Source: CAD feature listing. Evaluate the final solid. Frame: model axes, mm. A direction names the side the tool comes from. Give positions to 0.01 mm unless a question says otherwise; leave off trailing zeros. Loops run counter-clockwise (first coordinate to the right, second up) from the corner with the lowest first, then second, coordinate; pieces in that order, holes last. Notation, with made-up numbers: M 73,66 L 104,66 A10 ccw 104,78 Z; hole C 47,38 d8. An arc over 180 degrees is marked long. Put each result on its own line as item: value.
from build123d import *

# Parameters (mm, degrees)
SALIENTE_EXTRUIR1_DEPTH = 40
CORTAR_EXTRUIR4_DEPTH   = 10
CORTAR_EXTRUIR5_DEPTH   = 10
CORTAR_EXTRUIR6_DEPTH   = 2
CROQUIS8_R              = 1.5
CORTAR_EXTRUIR7_DEPTH   = 42
CROQUIS9_R              = 1.5
CORTAR_EXTRUIR8_DEPTH   = 42


with BuildPart() as part:
    # Croquis2 → Saliente-Extruir1 (new body)
    with BuildSketch(Plane.XY):
        Polygon((0, 26), (3, 26), (3, 4), (15, 4), (15, 0), (0, 0), align=None)
    extrude(amount=SALIENTE_EXTRUIR1_DEPTH)

    # Croquis6 → Cortar-Extruir4 (cut)
    with BuildSketch(Plane(origin=(3, 0, 0), x_dir=(0, 0, -1), z_dir=(1, 0, 0))):
        with BuildLine():
            Line((-40, 4), (-43.463242579, 10.305944429))
            Line((-43.463242579, 10.305944429), (-46.103119836, 28.990848346))
            Line((-46.103119836, 28.990848346), (-47.186653475, 36.660038985))
            Line((-47.186653475, 36.660038985), (8.796856155, 26.447825939))
            Line((8.796856155, 26.447825939), (6.381141064, 12.03440645))
            Line((6.381141064, 12.03440645), (0, 4))
            ThreePointArc((0, 4), (-20, 24), (-40, 4))
        make_face()
    extrude(amount=-CORTAR_EXTRUIR4_DEPTH, mode=Mode.SUBTRACT)

    # Croquis5 → Cortar-Extruir5 (cut)
    with BuildSketch(Plane(origin=(0, 4, 0), x_dir=(1, 0, 0), z_dir=(0, 1, 0))):
        with BuildLine():
            Line((15, -12), (15, -28))
            ThreePointArc((15, -28), (11.485281374, -36.485281374), (3, -40))
            Line((3, -40), (17.00840725, -44.81222058))
            Line((17.00840725, -44.81222058), (27.206798155, -5.039954665))
            Line((27.206798155, -5.039954665), (15.87267332, 7.755192399))
            Line((15.87267332, 7.755192399), (3, 0))
            ThreePointArc((3, 0), (11.485281374, -3.514718626), (15, -12))
        make_face()
    extrude(amount=-CORTAR_EXTRUIR5_DEPTH, mode=Mode.SUBTRACT)

    # Croquis7 → Cortar-Extruir6 (cut)
    with BuildSketch(Plane(origin=(0, 4, 0), x_dir=(1, 0, 0), z_dir=(0, 1, 0))):
        Polygon((7.9, -3.651368439), (5, -5.325684219), (5, -8.674315781), (7.9, -10.348631561), (10.8, -8.674315781), (10.8, -5.325684219), align=None)
        Polygon((5, -31.325684219), (5, -34.674315781), (7.9, -36.348631561), (10.8, -34.674315781), (10.8, -31.325684219), (7.9, -29.651368439), align=None)
    extrude(amount=-CORTAR_EXTRUIR6_DEPTH, mode=Mode.SUBTRACT)

    # Croquis8 → Cortar-Extruir7 (cut)
    with BuildSketch(Plane(origin=(0, 2, 0), x_dir=(1, 0, 0), z_dir=(0, 1, 0))):
        with Locations(Location((7.9, -7, 0), (0, 0, 270))):
            Circle(CROQUIS8_R)
    extrude(amount=-CORTAR_EXTRUIR7_DEPTH, mode=Mode.SUBTRACT)

    # Croquis9 → Cortar-Extruir8 (cut)
    with BuildSketch(Plane(origin=(0, 2, 0), x_dir=(1, 0, 0), z_dir=(0, 1, 0))):
        with Locations(Location((7.9, -33, 0), (0, 0, 180))):
            Circle(CROQUIS9_R)
    extrude(amount=-CORTAR_EXTRUIR8_DEPTH, mode=Mode.SUBTRACT)


solid = part.part
1. Section query B-B (z = 8). Output: boundary loops of the cut face in (x, y), plus the area to 3 significant figures.
Found:
outline: M 0,0 L 6.78,0 L 6.78,2 L 5,2 L 5,4 L 3,4 L 3,20 L 0,20 Z; M 9.02,0 L 14.31,0 L 14.31,4 L 10.8,4 L 10.8,2 L 9.02,2 Z
area: 89.2 mm^2
2. Section query A-A (y = 3.5). Output: boundary loops of the cut face in (x, z).
Found:
outline: M 0,0 L 3,0 A12 ccw 15,12 L 15,28 A12 ccw 3,40 L 0,40 Z; hole M 5,5.33 L 7.9,3.65 L 10.8,5.33 L 10.8,8.67 L 7.9,10.35 L 5,8.67 Z; hole M 5,31.33 L 7.9,29.65 L 10.8,31.33 L 10.8,34.67 L 7.9,36.35 L 5,34.67 Z
3. Draft query along Z for faces 4 (the flat face through (8, 0, 20)), 5 (the flat face through (9.37, 3.01, 30.5)), 6 (the cylindrical face through (11.58, 2.03, 36.39)). Return one class per face: pulls with the +Z half, pulls with the -Z half, needs draft (parallel to the pull), parting line crosses it, or undercut.
Found:
face 4: needs draft
face 5: undercut
face 6: pulls with the +Z half
4. Section query D-D (x = 6). Output: boundary loops of the cut face in (y, z), plus the area to 3 significant figures.
Found:
outline: M 0,0.38 L 4,0.38 L 4,4.75 L 2,4.75 L 2,9.25 L 4,9.25 L 4,30.75 L 2,30.75 L 2,35.25 L 4,35.25 L 4,39.62 L 0,39.62 Z
area: 139 mm^2
5. Section query C-C (y = 16). Output: boundary loops of the cut face in (x, z).
Found:
outline: M 0,4 L 3,4 L 3,36 L 0,36 Z
6. Contact query for flat-ended pins moving along their axis: P1, Ø6.5, axis at x = 7.5, z = 31.5, coming from the +Y side; P2, Ø1, axis at y = 3.5, z = 7.5, coming from the +X side; P3, Ø4, axis at x = 7.9, z = 33, coming from the +Y side; P4, Ø1.5, axis at x = 4, y = 18.5, coming from the -Z side. Output: stop coordinate, or through.
Found:
P1: y = 4
P2: x = 14.31
P3: y = 2
P4: through
7. Material intervals for line 1 (Y direction, x = 6.25, z = 31); line 2 (X direction, y = 2.5, z = 30); line 3 (X direction, y = 12, z = 35), sorted ascending. Write a range as from..to.
Found:
line 1: 0..2
line 2: 0..7.3, 8.5..14.83
line 3: 0..3
8. Access query for faces 1 (the flat face through (2, 2, 0)), 2 (the flat face through (6.47, 3.014, 30.477)), 3 (the flat face through (9, 4, 20)). Directions: +Z, -Z, +X, -X, +Y, -Y. A direction counts if a zero-diameter tool reaches every point of the face in a straight line with its end or side. Return the directions, or none.
Found:
face 1: -Z, +X, -X, +Y, -Y
face 2: +Y
face 3: +Z, -Z, +X, +Y
